Here's how the part is built. I have some questions about the finished solid (model axes, mm). Round coordinates to 2 decimals unless told otherwise and drop trailing zeros. Order: outer loops, then holes, each group sorted by start corner. A loop starts at its lowest first (then second) coordinate and runs counter-clockwise, first axis right, second up. Notation, with made-up numbers: M 17.5,-14.5 L 31.5,-14.5 A21 cw 31.5,20.5 Z; hole C 16,-19 d5. An arc over 180 degrees is marked long. Write item = value, one per line. Start each with the question number.
Item 1: I want a section at A-A, the plane z = -0.25. List the corners of the cut face in (x, y) for me, plus the area to 3 significant figures.
Item 2: Please list where these lines run through material, in increasing order: L1, parallel to X at y = 1, z = 0; L2, parallel to Y at x = -13.5, z = -0.7; L3, parallel to X at y = -1, z = -0.7.
Item 3: I want a section at B-B, the plane y = -3. List the corners of the cut face in (x, z) for me (1 decimal), plus the area to 3 significant figures.
Item 4: I'm going to push flat-ended pins straight in: P1, Ø5, axis at x = -10, y = 3, coming from the -Z side; P2, Ø2, axis at x = -6.5, y = 4, coming from the -Z side. Where does each tip first touch, or does it pass through?
```python
from build123d import *

# Parameters (mm, degrees)
SKETCH1_R = 0.9525


with BuildPart() as part:
    # Sweep1: sweep along a path in Sketch2
    with BuildLine(Plane.XY) as sweep1_path:
        Line((0, 3.683), (0, -3.683))
        ThreePointArc((0, -3.683), (-0.310403565, -4.514910261), (-1.089881388, -4.940162394))
        Line((-1.089881388, -4.940162394), (-17.278929773, -7.25963117))
        ThreePointArc((-17.278929773, -7.25963117), (-20.464864245, -6.322873659), (-21.844, -3.302))
        Line((-21.844, -3.302), (-21.844, 3.302))
        ThreePointArc((-21.844, 3.302), (-20.464864245, 6.322873659), (-17.278929773, 7.25963117))
        Line((-17.278929773, 7.25963117), (-1.089881388, 4.940162394))
        ThreePointArc((-1.089881388, 4.940162394), (-0.310403565, 4.514910261), (0, 3.683))
    # Sketch1 → Sweep1 (sweep)
    with BuildSketch(Plane(origin=(0, 0, 0), x_dir=(0, 0, -1), z_dir=(0, 1, 0))):
        Circle(SKETCH1_R)
    sweep(path=sweep1_path.line)


solid = part.part
```
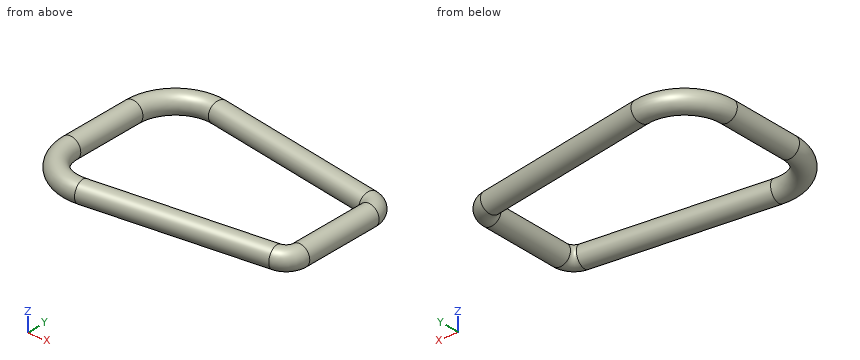
Filled in:
q1.outline = M -22.76,-3.3 A4.92 ccw -17.15,-8.17 L -0.96,-5.85 A2.19 ccw 0.92,-3.68 L 0.92,3.68 A2.19 ccw -0.96,5.85 L -17.15,8.17 A4.92 ccw -22.76,3.3 Z; hole M -20.92,-3.3 A3.08 ccw -17.41,-6.35 L -1.22,-4.03 A0.35 ccw -0.92,-3.68 L -0.92,3.68 A0.35 ccw -1.22,4.03 L -17.41,6.35 A3.08 ccw -20.92,3.3 Z
q1.area = 118 mm^2
q2.L1 = -22.8 to -20.89, -0.95 to 0.95
q2.L2 = -7.37 to -6.07, 6.07 to 7.37
q2.L3 = -22.49 to -21.2, -0.65 to 0.65
q3.outline = C -21.8,0 d1.9; C 0,0 d1.9
q3.area = 5.70 mm^2
q4.P1 = -0.66
q4.P2 = -0.65
